Model file for the job. Use its own axes, mm. A direction names the side the tool comes from. Round coordinates to 2 decimals unless told otherwise and drop trailing zeros. Loops run counter-clockwise (first coordinate to the right, second up) from the corner with the lowest first, then second, coordinate; pieces in that order, holes last. Notation, with made-up numbers: (-31.75, 69.25) -> (-23.75, 69.25) arc R31 cw to (-23.75, 95.25) -> close; hole circle Ø2 at (-15, -26). An arc over 180 degrees is marked (long way). Use a Markdown table: item, result. Add a question column.
```python
from build123d import *

# Parameters (mm, degrees)
SKETCH1_R                                      = 1.65
BOSS_EXTRUDE1_DEPTH                            = 3
SKETCH1_3_W                                    = 9
SKETCH1_3_H                                    = 2.5
BOSS_EXTRUDE2_DEPTH                            = 46.6
BOSS_EXTRUDE3_START                            = -49.6
SKETCH1_4_R                                    = 1.65
SKETCH1_4_W                                    = 9
SKETCH1_4_H                                    = 2.5
BOSS_EXTRUDE3_DEPTH                            = 3
CUT_EXTRUDE1_DEPTH                             = 88.5
SKETCH3_W                                      = 44.6
SKETCH3_H                                      = 2.5
BOSS_EXTRUDE4_DEPTH                            = 12
FILLET1_R                                      = 10
CSK_START                                      = -9
CSK_SLOT_FOR_M3_COUNTERSUNK_FLAT_HEAD_SC_DEPTH = 3


with BuildPart() as part:
    # Sketch1 → Boss-Extrude1 (new body)
    with BuildSketch(Plane.XY):
        Polygon((-13, 18.856406461), (-13, 11.696152423), (-4, 6.5), (-4, -9), (5, -9), (56, 30), (56, 42), (35.264699244, 42), (5, 18.856406461), align=None)
        Circle(SKETCH1_R, mode=Mode.SUBTRACT)
        with Locations((-8, 13.856406461)):
            Circle(SKETCH1_R, mode=Mode.SUBTRACT)
        with Locations((49, 36)):
            Circle(SKETCH1_R, mode=Mode.SUBTRACT)
        with Locations((39, 36)):
            Circle(SKETCH1_R, mode=Mode.SUBTRACT)
    extrude(amount=BOSS_EXTRUDE1_DEPTH)

    # Sketch1<3> → Boss-Extrude2 (add)
    with BuildSketch(Plane.XY):
        with Locations((0.5, -7.75)):
            Rectangle(SKETCH1_3_W, SKETCH1_3_H)
        Polygon((56, 33.77663551), (5, -6.5), (5, -9), (56, 30), align=None)
    extrude(amount=-BOSS_EXTRUDE2_DEPTH)

    # Sketch1<4> → Boss-Extrude3 (add)
    # profile 1 of 4: a face of its own
    with BuildSketch(Plane.XY.offset(BOSS_EXTRUDE3_START)):
        Polygon((5, 18.856406461), (-13, 18.856406461), (-13, 11.696152423), (-4, 6.5), (-4, -6.5), (5, -6.5), align=None)
        Circle(SKETCH1_4_R, mode=Mode.SUBTRACT)
        with Locations((-8, 13.856406461)):
            Circle(SKETCH1_4_R, mode=Mode.SUBTRACT)
    # profile 2 of 4: a face of its own
    with BuildSketch(Plane.XY.offset(BOSS_EXTRUDE3_START)):
        with Locations((0.5, -7.75)):
            Rectangle(SKETCH1_4_W, SKETCH1_4_H)
    # profile 3 of 4: a face of its own
    with BuildSketch(Plane.XY.offset(BOSS_EXTRUDE3_START)):
        Polygon((56, 33.77663551), (5, -6.5), (5, -9), (56, 30), align=None)
    # profile 4 of 4: a face of its own
    with BuildSketch(Plane.XY.offset(BOSS_EXTRUDE3_START)):
        Polygon((35.264699244, 42), (5, 18.856406461), (5, -6.5), (56, 33.77663551), (56, 42), align=None)
        with Locations((39, 36)):
            Circle(SKETCH1_4_R, mode=Mode.SUBTRACT)
        with Locations((49, 36)):
            Circle(SKETCH1_4_R, mode=Mode.SUBTRACT)
    extrude(amount=BOSS_EXTRUDE3_DEPTH)

    # Sketch2 → Cut-Extrude1 (cut)
    with BuildSketch(Plane.XZ.offset(9)):
        with BuildLine():
            Line((1, -24.95), (-1, -24.95))
            ThreePointArc((-1, -24.95), (-2.65, -23.3), (-1, -21.65))
            Line((-1, -21.65), (1, -21.65))
            ThreePointArc((1, -21.65), (2.65, -23.3), (1, -24.95))
        make_face()
    extrude(amount=-CUT_EXTRUDE1_DEPTH, mode=Mode.SUBTRACT)

    # Sketch3 → Boss-Extrude4 (add)
    with BuildSketch(Plane.ZY.offset(4)):
        with Locations((-23.3, -7.75)):
            Rectangle(SKETCH3_W, SKETCH3_H)
    extrude(amount=BOSS_EXTRUDE4_DEPTH)

    # Fillet1
    fillet1_edges = [part.edges().sort_by_distance(p)[0] for p in [
        (-16, -7.75, -45.6),
        (-16, -7.75, -1),
    ]]
    fillet(fillet1_edges, radius=FILLET1_R)

    # CSK SLOT for M3 Countersunk Flat Head Screw1: read off the stored shape, not the designer's step
    # CSK SLOT for M3 Countersunk Flat Hea 2 → CSK SLOT for M3 Countersunk Flat Head Screw1 (cut)
    with BuildSketch(Plane(origin=(0, 0, 0), x_dir=(1, 0, 0), z_dir=(0, 1, 0)).offset(CSK_START)):
        with BuildLine():
            ThreePointArc((1.7125, 24.788235112), (1.229705955, 25.020294045), (0.7, 25.1))
            Line((0.7, 25.1), (-0.7, 25.1))
            ThreePointArc((-0.7, 25.1), (-1.229705955, 25.020294045), (-1.7125, 24.788235112))
            ThreePointArc((-1.7125, 24.788235112), (-1.365316345, 24.909050642), (-1, 24.95))
            Line((-1, 24.95), (1, 24.95))
            ThreePointArc((1, 24.95), (1.365316345, 24.909050642), (1.7125, 24.788235112))
        make_face()
        with BuildLine():
            ThreePointArc((0.7, 21.5), (1.229705955, 21.579705955), (1.7125, 21.811764888))
            ThreePointArc((1.7125, 21.811764888), (1.365316345, 21.690949358), (1, 21.65))
            Line((1, 21.65), (-1, 21.65))
            ThreePointArc((-1, 21.65), (-1.365316345, 21.690949358), (-1.7125, 21.811764888))
            ThreePointArc((-1.7125, 21.811764888), (-1.229705955, 21.579705955), (-0.7, 21.5))
            Line((-0.7, 21.5), (0.7, 21.5))
        make_face()
    extrude(amount=CSK_SLOT_FOR_M3_COUNTERSUNK_FLAT_HEAD_SC_DEPTH, mode=Mode.SUBTRACT)

    # CSK SLOT for M3 Countersunk Flat Hea 3: loft between two sections, ruled curve by curve
    csk_slot_for_m3_countersunk_flat_hea_3_from = [
        Edge.make_three_point_arc((0.7, -7.649999999, -25.099999999), (1.972792205, -7.649999999, -24.572792205), (2.499999999, -7.649999999, -23.3)),
        Edge.make_three_point_arc((2.499999999, -7.649999999, -23.3), (1.972792205, -7.649999999, -22.027207795), (0.7, -7.649999999, -21.500000001)),
        Edge.make_three_point_arc((-0.7, -7.649999999, -21.500000001), (-1.972792205, -7.649999999, -22.027207795), (-2.499999999, -7.649999999, -23.3)),
        Edge.make_three_point_arc((-2.499999999, -7.649999999, -23.3), (-1.972792205, -7.649999999, -24.572792205), (-0.7, -7.649999999, -25.099999999)),
        Edge.make_line((0.7, -7.649999999, -21.500000001), (-0.7, -7.649999999, -21.500000001)),
        Edge.make_line((0.7, -7.649999999, -25.099999999), (-0.7, -7.649999999, -25.099999999)),
    ]
    csk_slot_for_m3_countersunk_flat_hea_3_to = [
        Edge.make_three_point_arc((0.7, -9, -26.45), (2.927386361, -9, -25.527386361), (3.85, -9, -23.3)),
        Edge.make_three_point_arc((3.85, -9, -23.3), (2.927386361, -9, -21.072613639), (0.7, -9, -20.15)),
        Edge.make_three_point_arc((-0.7, -9, -20.15), (-2.927386361, -9, -21.072613639), (-3.85, -9, -23.3)),
        Edge.make_three_point_arc((-3.85, -9, -23.3), (-2.927386361, -9, -25.527386361), (-0.7, -9, -26.45)),
        Edge.make_line((0.7, -9, -20.15), (-0.7, -9, -20.15)),
        Edge.make_line((0.7, -9, -26.45), (-0.7, -9, -26.45)),
    ]
    csk_slot_for_m3_countersunk_flat_hea_3 = Solid(Shell([*[Face.make_surface_from_curves(csk_slot_for_m3_countersunk_flat_hea_3_from[k], csk_slot_for_m3_countersunk_flat_hea_3_to[k]) for k in range(6)], Face(Wire(csk_slot_for_m3_countersunk_flat_hea_3_from)), Face(Wire(csk_slot_for_m3_countersunk_flat_hea_3_to))]))
    add(csk_slot_for_m3_countersunk_flat_hea_3, mode=Mode.SUBTRACT)


solid = part.part
```
1) Cut at C-C on y = 0. Write the cut outline in (x, z).
2) Cut at D-D on x = 18. Write the cut outline in (y, z), and give its area (3 significant figures).
3) Wall check: probe 1 along Y at (x, z) = (0, 1.2); probe 2 along Z at (x, y) = (24.5, 11); probe 3 along Y at (x, z) = (39, 0.6). Give the ranges that are in metal, low to high. Write a range as from..to.
4) Cut at A-A on y = 36. Write the cut outline in (x, z).
5) Tool access for faces 4 (the face through (21, 18, -46.6)), 5 (the face through (-4, 18.856, -48)), 6 (the face through (-4, -1, -48)): list every direction of +Z, -Z, +X, -X, +Y, -Y with a clear straight run to the whole face (end or side of a thin tool).
6) Pull direction Y, two halves, no side cores. Call faces 1 (the face through (-9.22, 14.97, 1.48)), 2 (the face through (-16, -8, -23)), 3 (the face through (-6, -9, -24)): +Y half, -Y half, draft (parallel to the pull), parting line (faces both ways), or undercut.
7) Cut at B-B on x = 39. Write the cut outline in (y, z).
8) Pin check, flat tips, straight feed: pin 1 Ø5 at (x, z) = (18.5, -11) entering from +Y; pin 2 Ø2.5 at (y, z) = (13.5, 1) entering from -X; pin 3 Ø3 at (x, y) = (49, 36) entering from -Z; pin 4 Ø1.5 at (x, z) = (8.5, -4.5) entering from -Y. Stop position of each tip, or through.
Established:
| question | item | result |
|---|---|---|
| 1 | outline | (-4, -49.6) -> (-1.65, -49.6) -> (-1.65, -46.6) -> (-4, -46.6) -> close; (-4, 0) -> (-1.65, 0) -> (-1.65, 3) -> (-4, 3) -> close; (1.65, -49.6) -> (16.77, -49.6) -> (16.77, 3) -> (1.65, 3) -> (1.65, 0) -> (13.23, 0) -> (13.23, -46.6) -> (1.65, -46.6) -> close |
| 2 | outline | (0.94, -49.6) -> (28.8, -49.6) -> (28.8, -46.6) -> (3.77, -46.6) -> (3.77, 0) -> (28.8, 0) -> (28.8, 3) -> (0.94, 3) -> close |
| 2 | area | 299 mm^2 |
| 3 | probe 1 | y = -9..-1.65, 1.65..18.86 |
| 3 | probe 2 | z = -49.6..-46.6, 0..3 |
| 3 | probe 3 | y = 17..34.35, 37.65..42 |
| 4 | outline | (27.42, -49.6) -> (37.35, -49.6) -> (37.35, -46.6) -> (27.42, -46.6) -> close; (27.42, 0) -> (37.35, 0) -> (37.35, 3) -> (27.42, 3) -> close; (40.65, -49.6) -> (47.35, -49.6) -> (47.35, -46.6) -> (40.65, -46.6) -> close; (40.65, 0) -> (47.35, 0) -> (47.35, 3) -> (40.65, 3) -> close; (50.65, -49.6) -> (56, -49.6) -> (56, -46.6) -> (50.65, -46.6) -> close; (50.65, 0) -> (56, 0) -> (56, 3) -> (50.65, 3) -> close |
| 5 | face 4 | -X, +Y |
| 5 | face 5 | +Z, -Z, -X, +Y |
| 5 | face 6 | -Z, -X, -Y |
| 6 | face 1 | undercut |
| 6 | face 2 | draft |
| 6 | face 3 | -Y half |
| 7 | outline | (17, -49.6) -> (34.35, -49.6) -> (34.35, -46.6) -> (20.35, -46.6) -> (20.35, 0) -> (34.35, 0) -> (34.35, 3) -> (17, 3) -> close; (37.65, -49.6) -> (42, -49.6) -> (42, -46.6) -> (37.65, -46.6) -> close; (37.65, 0) -> (42, 0) -> (42, 3) -> (37.65, 3) -> close |
| 8 | pin 1 | stops at y = 6.14 |
| 8 | pin 2 | stops at x = -13 |
| 8 | pin 3 | passes through |
| 8 | pin 4 | stops at y = -6.9 |
